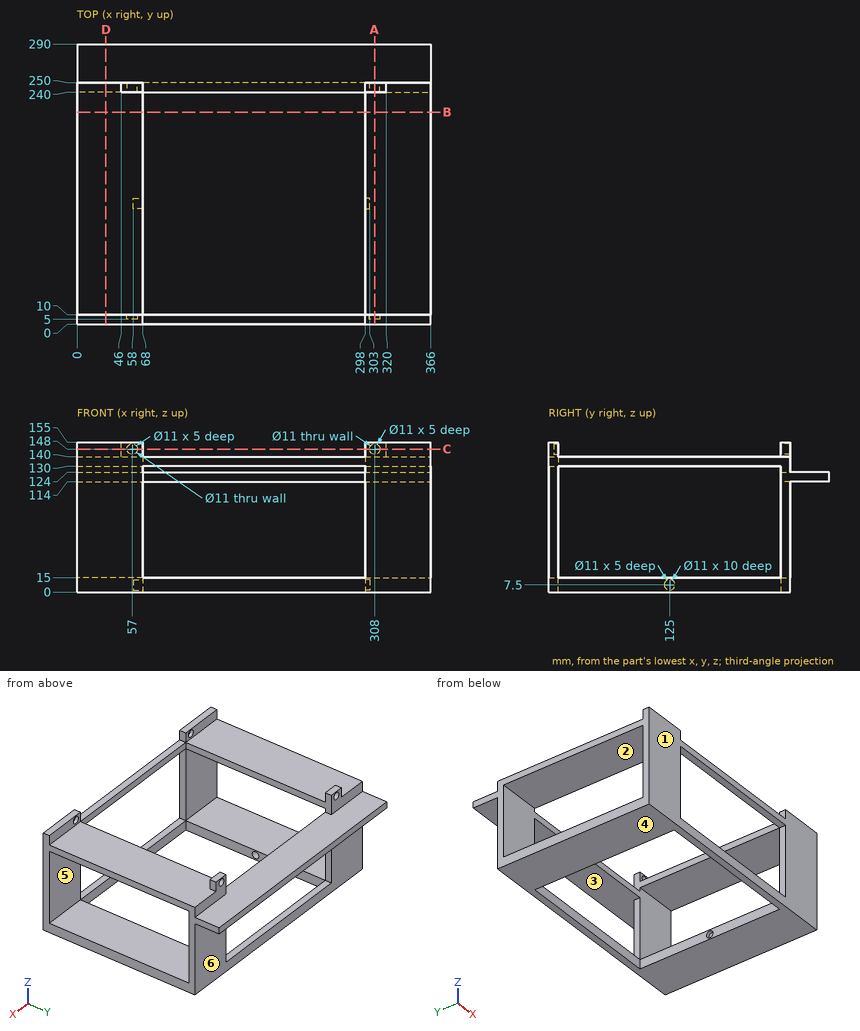
Verification items for this drawing (mm, ordinates from the low corner). A direction names the side the tool comes from. Give positions to 0.01 mm unless a question says otherwise; leave off trailing zeros. Loops run counter-clockwise (first coordinate to the right, second up) from the corner with the lowest first, then second, coordinate; pieces in that order, holes last.
(1) Release check for a two-part mould opening along Z. For the marked faces 4, 5 and 6 record: released by +Z, released by -Z, zero draft, split by the parting line, or undercut.
From the geometry:
face 4: released by -Z
face 5: undercut
face 6: zero draft
(2) Depth check by flat-ended pin: pin 1 Ø12 at (x, z) = (45, 145) entering from +Y; pin 2 Ø3.5 at (x, z) = (54.5, 147.5) entering from +Y; pin 3 Ø6 at (x, y) = (40.5, 244.5) entering from +Z. Enter the tip coordinate at first touch or a pass-through.
From the geometry:
pin 1: stops at y = 250
pin 2: stops at y = 5
pin 3: stops at z = 140
(3) Section check B-B on y = 219.5. Record the cut outline in (x, z).
From the geometry:
outline: (0, 0) - (68, 0) - (68, 15) - (0, 15) - close; (0, 130) - (68, 130) - (68, 140) - (0, 140) - close; (298, 0) - (366, 0) - (366, 15) - (298, 15) - close; (298, 130) - (366, 130) - (366, 140) - (298, 140) - close
(4) Thickness scan on L1, parallel to Z at x = 64.75, y = 125; L2, parallel to X at y = 8.55, z = 148; L3, parallel to Z at x = 310, y = 176. Record the ranges inside material, lowest first.
From the geometry:
L1: z = 0 to 2, 13 to 15, 130 to 140
L2: x = 0 to 51.5, 62.5 to 68, 298 to 302.5, 313.5 to 366
L3: z = 0 to 15, 130 to 140
(5) Section check C-C on z = 148. Count the separate pieces of the cut face and the enclosed holes in it, then the cut area to 3 significant figures.
From the geometry:
separate pieces: 6
enclosed holes: 0
area: 1,470 mm2
(6) Section check D-D on x = 30. Record the cut outline in (y, z), then the cut area to 3 significant figures.
From the geometry:
outline: (0, 0) - (250, 0) - (250, 114) - (290, 114) - (290, 124) - (250, 124) - (250, 140) - (10, 140) - (10, 155) - (0, 155) - close; hole (10, 15) - (240, 15) - (240, 130) - (10, 130) - close
area: 9,100 mm2
(7) Section check A-A on x = 308. Record the cut outline in (y, z), then the cut area to 4 significant figures.
From the geometry:
outline: (0, 0) - (250, 0) - (250, 114) - (290, 114) - (290, 124) - (250, 124) - (250, 142.5) - (240, 142.5) - (240, 140) - (10, 140) - (10, 142.5) - (5, 142.5) - (5, 153.5) - (10, 153.5) - (10, 155) - (0, 155) - close; (240, 153.5) - (250, 153.5) - (250, 155) - (240, 155) - close; hole (10, 15) - (240, 15) - (240, 130) - (10, 130) - close
area: 9,085 mm2
(8) Set-up check for the marked faces 1, 2 and 3: record each of +Z, -Z, +X, -X, +Y, -Y from which the full face is reachable in a straight line by a thin tool's end or side.
From the geometry:
face 1: +Z, -Z, +X, -X, -Y
face 2: +X, -X
face 3: +Y
